from build123d import *

# Parameters (mm, degrees)
BOSS_EXTRUDE1_DEPTH      = 12.7
BOSS_EXTRUDE1_DEPTH_BACK = 12.7
SKETCH1_W                = 76.2
SKETCH1_H                = 25.4
CUT_EXTRUDE1_DEPTH       = 48.519048812
SKETCH4_R                = 7.9375
BOSS_EXTRUDE2_DEPTH      = 76.2
BOSS_EXTRUDE3_DEPTH      = 10
BOSS_EXTRUDE5_DEPTH      = 7.178167


with BuildPart() as part:
    # Sketch1 → Boss-Extrude1 (new, two sides: drawn at the far end of the back side and taken through both)
    with BuildSketch(Plane.XY.offset(-BOSS_EXTRUDE1_DEPTH_BACK)):
        Rectangle(SKETCH1_W, SKETCH1_H)
    extrude(amount=BOSS_EXTRUDE1_DEPTH + BOSS_EXTRUDE1_DEPTH_BACK)

    # Sketch2 → Cut-Extrude1 (cut, through all)
    with BuildSketch(Plane.XZ.offset(12.7)):
        Polygon((34.199985956, 0), (30.299971912, -12.7), (38.1, -12.7), (38.1, -1.197646421), align=None)
        Polygon((38.1, 12.7), (34.199985956, 0), (38.1, -1.197646421), align=None)
        with BuildLine():
            Line((30.299971912, -12.7), (-38.1, -12.7))
            Line((-38.1, -12.7), (-38.1, 2.7))
            Line((-38.1, 2.7), (-9.105646135, 2.7))
            add(Edge.make_bspline(
                [(30.299971912, -12.7), (25.466803171, -12.7), (16.707798139, -8.78817181), (4.449206283, -1.21182819), (-4.185142014, 2.7), (-9.105646135, 2.7)],
                knots=[0, 0, 0, 0, 0.311689084, 0.688310916, 1, 1, 1, 1], degree=3))
        make_face()
    extrude(amount=-CUT_EXTRUDE1_DEPTH, mode=Mode.SUBTRACT)

    # Sketch4 → Boss-Extrude2 (add)
    with BuildSketch(Plane(origin=(31.252760971, 0, -9.59733911), x_dir=(-0.2935578385035089, 0, -0.95594131381228), z_dir=(0.95594131381228, 0, -0.2935578385035089))):
        with Locations((-10.039678032, 0)):
            Circle(SKETCH4_R)
    extrude(amount=BOSS_EXTRUDE2_DEPTH)

    # Sketch5 → Boss-Extrude3 (add)
    with BuildSketch(Plane(origin=(0, 0, 2.7), x_dir=(-1, 0, 0), z_dir=(0, 0, -1))):
        Polygon((9.105646135, -12.7), (27.661608652, -26.617413502), (38.1, -12.7), align=None)
        Polygon((38.1, -12.7), (57.150604496, 12.7), (38.1, 12.7), align=None)
    extrude(amount=-BOSS_EXTRUDE3_DEPTH)

    # Sketch7 → Boss-Extrude5 (add)
    with BuildSketch(Plane.XY.offset(12.7)):
        Polygon((-57.150604496, 12.7), (-27.661608652, -26.617413502), (-9.105646135, -12.7), (38.1, -12.7), (38.1, 12.7), align=None)
    extrude(amount=BOSS_EXTRUDE5_DEPTH)


solid = part.part
Input: part model. Units: mm. Frame: model coordinates. A direction names the side the tool comes from. Give positions to 0.01 mm unless a question says otherwise; leave off trailing zeros. Write each loop counter-clockwise with the first axis right and the second up, starting at its lowest first coordinate (ties: lowest second). Pieces come first, ordered by that corner, then holes.
Q1. Section C-C, the plane x = -14. Output: boundary loops of the cut face in (y, z).
Q2. Pull-direction query (X, two-part tool) for faces 1 (the face through (-9, 12.7, 7)), 2 (the face through (107.075, 0.111, -22.263)), 3 (the face through (35.988, -5.822, 5.822)); classes: pulls with the +X half, pulls with the -X half, needs draft (parallel to the pull), parting line crosses it, or undercut.
Q3. Material intervals for probe 1 along Y at (x, z) = (33.5, 4); probe 2 along Z at (x, y) = (-24.5, -23); probe 3 along Z at (x, y) = (14, -10), sorted ascending.
Q4. Section B-B, the plane y = -18. Output: boundary loops of the cut face in (x, z), plus the area to 3 significant figures.
Q5. First-contact query: P1, Ø6, axis at y = -10, z = 7.5, coming from the -X side; P2, Ø10, axis at x = 16, z = 1.5, coming from the -Y side; P3, Ø12, axis at x = -42.5, y = -10.5, coming from the -Z side. Flat tips, straight axial feed; report the tip coordinate or a pass-through.
Q6. Set-up query: faces 4 (the face through (-10, -2, 19.878)), 5 (the face through (70.617, -7.749, -9.383)), 6 (the face through (14, -12.7, 7)), 7 (the face through (-27, -2, 2.7)), 8 (the face through (38.1, 0, 16)). Return all of +Z, -Z, +X, -X, +Y, -Y with unobstructed straight access to the full face (end or side cutting, diameter ignored); none if empty.
Q7. Section A-A, the plane x = -32. Output: boundary loops of the cut face in (y, z), plus the area to 3 significant figures.
Filled in:
1. outline: (-16.37, 2.7) - (12.7, 2.7) - (12.7, 19.88) - (-16.37, 19.88) - close
2. face 1: needs draft
2. face 2: pulls with the +X half
2. face 3: undercut
3. probe 1: y = -12.7 to 12.7
3. probe 2: z = 2.7 to 19.88
3. probe 3: z = -6.94 to 19.88
4. outline: (-34.12, 2.7) - (-16.17, 2.7) - (-16.17, 19.88) - (-34.12, 19.88) - close
4. area: 308 mm2
5. P1: stops at x = -42.38
5. P2: stops at y = -12.7
5. P3: stops at z = 2.7
6. face 4: +Z, +X, -X, +Y, -Y
6. face 5: none
6. face 6: +Z, -Z, +X, -Y
6. face 7: -Z, -X, +Y, -Y
6. face 8: +Z, +X, +Y, -Y
7. outline: (-20.83, 2.7) - (12.7, 2.7) - (12.7, 19.88) - (-20.83, 19.88) - close
7. area: 576 mm2
